from build123d import *

# Parameters (mm, degrees)
SKETCH1_W                             = 88.9
SKETCH1_H                             = 304.8
SKETCH1_W_2                           = 63.5
SKETCH1_H_2                           = 254
BOSS_EXTRUDE1_DEPTH                   = 3.175
SKETCH7_R                             = 2.159
CUT_EXTRUDE2_DEPTH                    = 159.781746826
FILLET1_R                             = 12.7
FILLET3_R                             = 3.175
SKETCH9_R                             = 2.159
CUT_EXTRUDE4_DEPTH                    = 159.781746826
SKETCH10_R                            = 2.38125
SONAR_HOLES_DEPTH                     = 159.781746826
SKETCH11_R                            = 2.38125
SONAR_HOLES_2_ELECTRIC_BOOGALOO_DEPTH = 159.781746826


with BuildPart() as part:
    # Sketch1 → Boss-Extrude1 (new body)
    with BuildSketch(Plane(origin=(0, 0, 0), x_dir=(1, 0, 0), z_dir=(0, 1, 0))):
        Rectangle(SKETCH1_W, SKETCH1_H)
        with Locations((0, -1.176932577)):
            Rectangle(SKETCH1_W_2, SKETCH1_H_2, mode=Mode.SUBTRACT)
    extrude(amount=BOSS_EXTRUDE1_DEPTH)

    # Sketch7 → Cut-Extrude2 (cut, through all)
    with BuildSketch(Plane(origin=(0, 3.175, 0), x_dir=(1, 0, 0), z_dir=(0, 1, 0))):
        with Locations(Location((-38.1, 139.736298381, 0), (0, 0, 270))):
            Circle(SKETCH7_R)
        with Locations(Location((38.1, 139.736298381, 0), (0, 0, 90))):
            Circle(SKETCH7_R)
        with Locations(Location((-38.1, 46.602880381, 0), (0, 0, 270))):
            Circle(SKETCH7_R)
        with Locations(Location((-38.1, -46.530537619, 0), (0, 0, 270))):
            Circle(SKETCH7_R)
        with Locations(Location((-38.1, -139.663955619, 0), (0, 0, 270))):
            Circle(SKETCH7_R)
        with Locations(Location((38.1, 46.602118381, 0), (0, 0, 90))):
            Circle(SKETCH7_R)
        with Locations(Location((38.1, -46.532061619, 0), (0, 0, 90))):
            Circle(SKETCH7_R)
        with Locations(Location((38.1, -139.666241619, 0), (0, 0, 90))):
            Circle(SKETCH7_R)
    extrude(amount=-CUT_EXTRUDE2_DEPTH, mode=Mode.SUBTRACT)

    # Fillet1
    fillet1_edges = [part.edges().sort_by_distance(p)[0] for p in [
        (-31.75, 1.5875, -125.823067423),
        (-31.75, 1.5875, 128.176932577),
        (31.75, 1.5875, 128.176932577),
        (31.75, 1.5875, -125.823067423),
    ]]
    fillet(fillet1_edges, radius=FILLET1_R)

    # Fillet3
    fillet3_edges = [part.edges().sort_by_distance(p)[0] for p in [
        (-44.45, 1.5875, -152.4),
        (44.45, 1.5875, -152.4),
        (44.45, 1.5875, 152.4),
        (-44.45, 1.5875, 152.4),
    ]]
    fillet(fillet3_edges, radius=FILLET3_R)

    # Sketch9 → Cut-Extrude4 (cut, through all)
    with BuildSketch(Plane(origin=(0, 3.175, 0), x_dir=(1, 0, 0), z_dir=(0, 1, 0))):
        with Locations(Location((-15.4178, 139.7, 0), (0, 0, 270))):
            Circle(SKETCH9_R)
        with Locations(Location((27.5844, 139.7, 0), (0, 0, 270))):
            Circle(SKETCH9_R)
    extrude(amount=-CUT_EXTRUDE4_DEPTH, mode=Mode.SUBTRACT)

    # Sketch10 → Sonar Holes (cut, through all)
    with BuildSketch(Plane(origin=(0, 3.175, 0), x_dir=(1, 0, 0), z_dir=(0, 1, 0))):
        with Locations(Location((-5.246249985, -132.458232577, 0), (0, 0, 270))):
            Circle(SKETCH10_R)
        with Locations(Location((5.246249985, -132.458232577, 0), (0, 0, 90))):
            Circle(SKETCH10_R)
    extrude(amount=-SONAR_HOLES_DEPTH, mode=Mode.SUBTRACT)

    # Sketch11 → Sonar Holes 2: Electric Boogaloo (cut, through all)
    with BuildSketch(Plane(origin=(0, 3.175, 0), x_dir=(1, 0, 0), z_dir=(0, 1, 0))):
        with Locations(Location((-38.181117115, 5.24625, 0), (0, 0, 270))):
            Circle(SKETCH11_R)
        with Locations(Location((-38.181117115, -5.24625, 0), (0, 0, 90))):
            Circle(SKETCH11_R)
        with Locations(Location((38.181117115, -5.24625, 0), (0, 0, 270))):
            Circle(SKETCH11_R)
        with Locations(Location((38.181117115, 5.24625, 0), (0, 0, 90))):
            Circle(SKETCH11_R)
    extrude(amount=-SONAR_HOLES_2_ELECTRIC_BOOGALOO_DEPTH, mode=Mode.SUBTRACT)


solid = part.part
Design review of the part built by this model. Coordinates are the model's own, in mm. A direction names the side the tool comes from. Round coordinates to 2 decimals unless told otherwise and drop trailing zeros. Use one line per item in the form item = value. Start each with the question number.
Q1. Draft analysis for pull direction X (two halves, no side actions). For faces 1 (the face through (27.931, 1.61, 124.555)), 2 (the face through (39, 3.175, -2)), 3 (the face through (-27.931, 1.61, 124.555)), state which applies: +X half, -X half, draft (parallel to the pull), parting line (faces both ways), or undercut.
Q2. We need section A-A on y = 0.8. State how many separate pieces and enclosed holes the cut face has, then the cut area to 3 significant figures.
Q3. Machinability: for faces 4 (the face through (39, 0, -2)), 5 (the face through (28.13, 1.61, -122)), which of the approach directions +Z, -Z, +X, -X, +Y, -Y give a long, thin tool a straight path to every point of the face, cutting with its end or side? Answer none if there is none.
Q4. Wall thickness on line 1 along Z through (x, y) = (-5.5, 0.6); line 2 along X through (y, z) = (2, -30); line 3 along Z through (x, y) = (6.5, 2.7): over which ranges is each line inside the solid? List them lowest first. Write a range as [from, to].
Calculated:
q1.face_1 = undercut
q1.face_2 = draft
q1.face_3 = undercut
q2.separate_pieces = 1
q2.enclosed_holes = 17
q2.area = 10,800 mm²
q3.face_4 = +Z, -Z, +X, -X, -Y
q3.face_5 = +Y, -Y
q4.line_1 = [-152.4, -125.82], [128.18, 130.09], [134.83, 152.4]
q4.line_2 = [-44.45, -31.75], [31.75, 44.45]
q4.line_3 = [-152.4, -125.82], [128.18, 130.43], [134.48, 152.4]
